For this review, take the finished solid that the model builds, in its own axes (mm). Give positions to 0.01 mm unless a question says otherwise; leave off trailing zeros. Order: outer loops, then holes, each group sorted by start corner. A loop starts at its lowest first (then second) coordinate and runs counter-clockwise, first axis right, second up. Notation, with made-up numbers: (9, 11.25) - (26, 11.25) arc R10 cw to (26, 15.25) - close; hole circle Ø2 at (17, -34). An arc over 180 degrees is marked (long way). Use a Markdown table: item, result. Add a question column.
1) We need section A-A on x = 0. Write out the cut boundary in (y, z), then the cut area to 3 significant figures.
2) Wall thickness on L1, parallel to Z at x = 0, y = 1.85; L2, parallel to X at y = -1.2, z = 13.5; L3, parallel to Z at x = 0.4, y = -0.1: over which ranges is each line inside the solid? List them lowest first.
3) Clearance check with flat-ended pins moving along their axes: P1, Ø1.9, axis at x = 0, z = 13.5, coming from the +Y side; P2, Ø1.5, axis at x = -0.5, z = -5.5, coming from the -Y side. State where each tip first meets the part, or that it passes through.
4) We need section C-C on z = 9.5. Write out the cut boundary in (x, y), then the cut area to 3 significant figures.
5) We need section B-B on z = 13.5. Write out the cut boundary in (x, y), then the cut area to 3 significant figures.
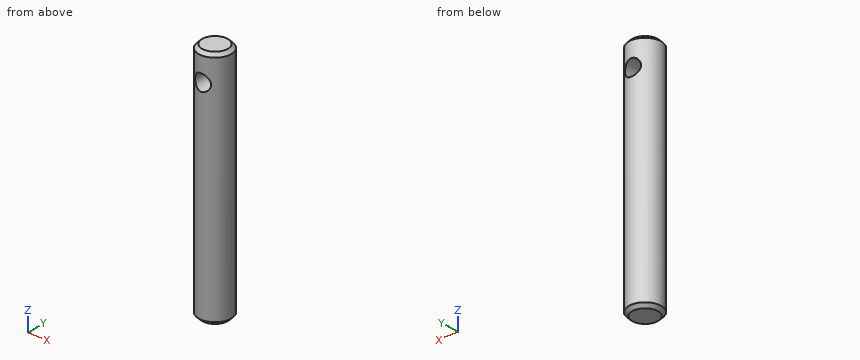
```python
from build123d import *

# Parameters (mm, degrees)
SKETCH1_R               = 2.38125
BOSS_EXTRUDE1_DEPTH     = 17.5
SKETCH2_R               = 1.190625
CUT_EXTRUDE2_DEPTH      = 3.38125
CUT_EXTRUDE2_DEPTH_BACK = 3.38125
CHAMFER1_SIZE           = 0.5


with BuildPart() as part:
    # Sketch1 → Boss-Extrude1 (new body, symmetric)
    with BuildSketch(Plane.XY):
        Circle(SKETCH1_R)
    extrude(amount=BOSS_EXTRUDE1_DEPTH, both=True)

    # Sketch2 → Cut-Extrude2 (cut, two sides)
    with BuildSketch(Plane(origin=(0, 0, 0), x_dir=(1, 0, 0), z_dir=(0, 1, 0))) as cut_extrude2_sk:
        with Locations((0, -13.5)):
            Circle(SKETCH2_R)
    extrude(amount=CUT_EXTRUDE2_DEPTH, mode=Mode.SUBTRACT)
    extrude(cut_extrude2_sk.sketch, amount=-CUT_EXTRUDE2_DEPTH_BACK, mode=Mode.SUBTRACT)

    # Chamfer1
    chamfer1_edges = [part.edges().sort_by_distance(p)[0] for p in [
        (-2.38125, 0, -17.5),
        (-2.38125, 0, 17.5),
    ]]
    chamfer(chamfer1_edges, length=CHAMFER1_SIZE)


solid = part.part
```
Checked values:
| question | item | result |
|---|---|---|
| 1 | outline | (-2.38, -17) - (-1.88, -17.5) - (1.88, -17.5) - (2.38, -17) - (2.38, 12.31) - (-2.38, 12.31) - close; (-2.38, 14.69) - (2.38, 14.69) - (2.38, 17) - (1.88, 17.5) - (-1.88, 17.5) - (-2.38, 17) - close |
| 1 | area | 155 mm² |
| 2 | L1 | -17.5 to 12.31, 14.69 to 17.5 |
| 2 | L2 | -2.06 to -1.19, 1.19 to 2.06 |
| 2 | L3 | -17.5 to 12.38, 14.62 to 17.5 |
| 3 | P1 | through |
| 3 | P2 | y = -2.38 |
| 4 | outline | circle Ø4.76 at (0, 0) |
| 4 | area | 17.8 mm² |
| 5 | outline | (-1.19, -2.06) - (-1.19, 2.06) arc R2.38 ccw to start; (1.19, -2.06) arc R2.38 ccw to (1.19, 2.06) - close |
| 5 | area | 6.97 mm² |
